Geometry: final body of the model. Coordinates: model frame, mm. Face numbers are marked on the shaded views. A direction names the side the tool comes from. Coordinates: 2 decimals unless noted, no trailing zeros. Write each loop counter-clockwise with the first axis right and the second up, starting at its lowest first coordinate (ties: lowest second). Pieces come first, ordered by that corner, then holes. Notation, with made-up numbers: (86, 28) - (112, 28) arc R20 cw to (112, 36) - close; hole circle Ø3 at (-38.5, 37). An arc over 180 degrees is marked (long way). Put each result on its own line as item: value.
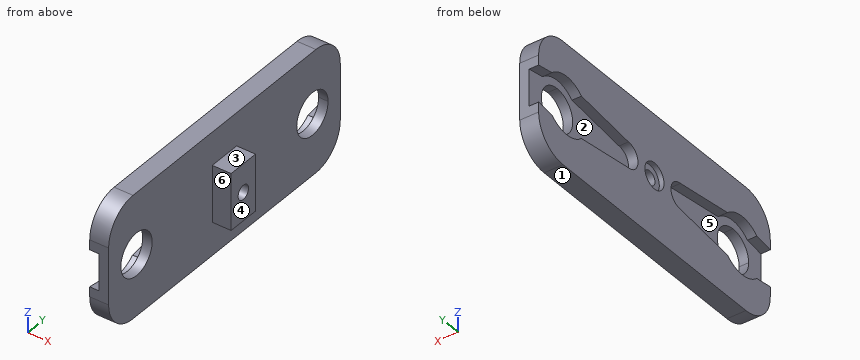
```python
from build123d import *

# Parameters (mm, degrees)
SKETCH_1_W             = 36.75
SKETCH_1_H             = 26
EXTRUDE_1_DEPTH        = 4
CUT_EXTRUDE_1_DEPTH    = 2
FILLET_1_R             = 7
CUT_EXTRUDE_3_DEPTH    = 2
SKETCH_11_W            = 12
SKETCH_11_H            = 7
EXTRUDE_2_DEPTH        = 4
SKETCH_12_R            = 1.5
CUT_EXTRUDE_4_DEPTH    = 8
SKETCH_13_R            = 2.75
CUT_EXTRUDE_5_DEPTH    = 1
FILLET_1_OF_MIRROR_2_R = 7


with BuildPart() as part:
    # Эскиз1 → Бобышка-Вытянуть1 (new body)
    with BuildSketch(Plane(origin=(0, 0, 0), x_dir=(0, -1, 0), z_dir=(-1, 0, 0))):
        with Locations((-0.875, 0)):
            Rectangle(SKETCH_1_W, SKETCH_1_H)
    extrude_1 = extrude(amount=-EXTRUDE_1_DEPTH)

    # Эскиз2 → Вырез-Вытянуть1 (cut)
    with BuildSketch(Plane.ZY):
        with BuildLine():
            Line((3.901238196, -17.5), (4.545454545, -13.652408939))
            ThreePointArc((4.545454545, -13.652408939), (6.222727273, -9.431365141), (4.545454545, -5.210321344))
            Line((4.545454545, -5.210321344), (2.795454545, 8.289678656))
            ThreePointArc((2.795454545, 8.289678656), (0.072727273, 11.012405929), (-2.65, 8.289678656))
            Line((-2.65, 8.289678656), (-4.4, -5.210321344))
            ThreePointArc((-4.4, -5.210321344), (-6.077272727, -9.431365141), (-4.4, -13.652408939))
            Line((-4.4, -13.652408939), (-3.901238196, -17.5))
            Line((-3.901238196, -17.5), (3.901238196, -17.5))
        make_face()
    cut_extrude_1 = extrude(amount=-CUT_EXTRUDE_1_DEPTH, mode=Mode.SUBTRACT)

    # Скругление1
    fillet_1_edges = [part.edges().sort_by_distance(p)[0] for p in [
        (2, -17.5, 13),
        (2, -17.5, -13),
    ]]
    fillet(fillet_1_edges, radius=FILLET_1_R)

    # Эскиз9 → Вырез-Вытянуть3 (cut)
    with BuildSketch(Plane.ZY.offset(-2)):
        with BuildLine():
            ThreePointArc((4.5, -9.5), (-3.181980515, -6.318019485), (0, -14))
            Line((0, -14), (0, -9.5))
            Line((0, -9.5), (4.5, -9.5))
        make_face()
        with BuildLine():
            Line((0, -9.5), (0, -14))
            ThreePointArc((0, -14), (3.181980515, -12.681980515), (4.5, -9.5))
            Line((4.5, -9.5), (0, -9.5))
        make_face()
    cut_extrude_3 = extrude(amount=-CUT_EXTRUDE_3_DEPTH, mode=Mode.SUBTRACT)

    # Эскиз11 → Бобышка-Вытянуть2 (add)
    with BuildSketch(Plane(origin=(4, 0, 0), x_dir=(0, 0, -1), z_dir=(1, 0, 0))):
        with Locations((0, 15.75)):
            Rectangle(SKETCH_11_W, SKETCH_11_H)
    extrude_2 = extrude(amount=EXTRUDE_2_DEPTH)

    # Эскиз12 → Вырез-Вытянуть4 (cut)
    with BuildSketch(Plane.ZY):
        with Locations((0, 15.75)):
            Circle(SKETCH_12_R)
    cut_extrude_4 = extrude(amount=-CUT_EXTRUDE_4_DEPTH, mode=Mode.SUBTRACT)

    # Эскиз13 → Вырез-Вытянуть5 (cut)
    with BuildSketch(Plane.ZY):
        with Locations((0, 15.75)):
            Circle(SKETCH_13_R)
    cut_extrude_5 = extrude(amount=-CUT_EXTRUDE_5_DEPTH, mode=Mode.SUBTRACT)

    # Зеркальное отражение2: Бобышка-Вытянуть1, Вырез-Вытянуть1, Вырез-Вытянуть3, Бобышка-Вытянуть2, Вырез-Вытянуть4, Вырез-Вытянуть5 across plane
    add(extrude_1.mirror(Plane.ZX.offset(15.75)))
    add(cut_extrude_1.mirror(Plane.ZX.offset(15.75)), mode=Mode.SUBTRACT)
    add(cut_extrude_3.mirror(Plane.ZX.offset(15.75)), mode=Mode.SUBTRACT)
    add(extrude_2.mirror(Plane.ZX.offset(15.75)))
    add(cut_extrude_4.mirror(Plane.ZX.offset(15.75)), mode=Mode.SUBTRACT)
    add(cut_extrude_5.mirror(Plane.ZX.offset(15.75)), mode=Mode.SUBTRACT)

    # Скругление1 of Зеркальное отражение2
    fillet_1_of_mirror_2_edges = [part.edges().sort_by_distance(p)[0] for p in [
        (2, 49, 13),
        (2, 49, -13),
    ]]
    fillet(fillet_1_of_mirror_2_edges, radius=FILLET_1_OF_MIRROR_2_R)


solid = part.part
```
1. Pin query (flat end, axial travel): pin 1 Ø1.6 at (y, z) = (16.5, 1.5) entering from -X; pin 2 Ø12 at (y, z) = (26, 5) entering from +X; pin 3 Ø6 at (y, z) = (40.5, 0) entering from -X; pin 4 Ø2 at (x, z) = (6, 1) entering from +Y. Return the tip coordinate at first contact, or that it passes through.
Answer below:
pin 1: stops at x = 1
pin 2: stops at x = 4
pin 3: passes through
pin 4: stops at y = 19.25
2. Section query B-B (y = 15.75). Return loops of the section in (x, z).
Answer below:
outline: (0, -13) - (4, -13) - (4, -6) - (8, -6) - (8, -1.5) - (1, -1.5) - (1, -2.75) - (0, -2.75) - close; (0, 2.75) - (1, 2.75) - (1, 1.5) - (8, 1.5) - (8, 6) - (4, 6) - (4, 13) - (0, 13) - close
3. Section query D-D (y = -4). Return loops of the section in (x, z), then the cut area to 3 significant figures.
Answer below:
outline: (0, -13) - (4, -13) - (4, 13) - (0, 13) - (0, 4.39) - (2, 4.39) - (2, -4.24) - (0, -4.24) - close
area: 86.7 mm²
4. Set-up query: the marked faces 4, 5 and 6. Return all of +Z, -Z, +X, -X, +Y, -Y with unobstructed straight access to the full face (end or side cutting, diameter ignored); none if empty.
Answer below:
face 4: +Z, -Z, +X, +Y, -Y
face 5: -X
face 6: +Z, -Z, +X, -Y
5. Mould query, pull axis Z, two halves, no side actions, for the marked faces 1, 2 and 3. Classes: +Z half, -Z half, draft (parallel to the pull), parting line (faces both ways), or undercut.
Answer below:
face 1: -Z half
face 2: undercut
face 3: +Z half
6. Section query A-A (x = 3.25). Return loops of the section in (y, z), then the cut area to 3 significant figures.
Answer below:
outline: (-17.5, -6) arc R7 ccw to (-10.5, -13) - (42, -13) arc R7 ccw to (49, -6) - (49, 6) arc R7 ccw to (42, 13) - (-10.5, 13) arc R7 ccw to (-17.5, 6) - close; hole circle Ø9 at (-9.5, 0); hole circle Ø3 at (15.75, 0); hole circle Ø9 at (41, 0)
area: 1,550 mm²
7. Section query C-C (x = 6.75). Return loops of the section in (y, z), then the cut area to 3 significant figures.
Answer below:
outline: (12.25, -6) - (19.25, -6) - (19.25, 6) - (12.25, 6) - close; hole circle Ø3 at (15.75, 0)
area: 76.9 mm²
8. Ray query, probe 1 along Z at (x, y) = (2.8, -9.5); probe 2 along Y at (x, z) = (3.75, 0.25); probe 3 along Z at (x, y) = (0.7, 15.75). Return the intervals inside material, ascending. Write a range as from..to.
Answer below:
probe 1: z = -13..-4.5, 4.5..13
probe 2: y = -17.5..-13.99, -5.01..14.27, 17.23..36.51, 45.49..49
probe 3: z = -13..-2.75, 2.75..13
